Verification items for the finished model (mm, model axes). Coordinates: 2 decimals unless noted, no trailing zeros. Order: outer loops, then holes, each group sorted by start corner. A loop starts at its lowest first (then second) coordinate and runs counter-clockwise, first axis right, second up.
Q1. Depth check by flat-ended pin: P1, Ø8, axis at x = 25, z = 30, coming from the -Y side. Enter the tip coordinate at first touch or a pass-through.
Q2. Draft check along X on faces 1 (the flat face through (30, -2, 81)), 2 (the cylindrical face through (46.15, -1.01, 67.78)). Enter one of: pulls with the +X half, pulls with the -X half, needs draft (parallel to the pull), parting line crosses it, or undercut.
Q3. Cross-section at B-B, the plane z = 150. Record the boundary of the cut face in (x, y).
Q4. Cross-section at C-C, the plane y = -0.7. Count the separate pieces of the cut face and the enclosed holes in it, and give its area (3 significant figures).
Q5. Cross-section at A-A, the plane x = 35. Record the boundary of the cut face in (y, z), and give its area (3 significant figures).
Q6. Thickness scan on line 1 (Z direction, x = 5, y = -0.85); line 2 (Z direction, x = 15, y = -0.55). Record the ranges inside material, lowest first.
from build123d import *

# Parameters (mm, degrees)
SKETCH_W                     = 60
SKETCH_H                     = 160
PAD_DEPTH                    = 2
SKETCH001_R                  = 2.5
POCKET_DEPTH                 = 343.784557
SKETCH001_LINEARPATTERN_2_R  = 2.5
POCKET_LINEARPATTERN_2_DEPTH = 343.784557
SKETCH001_LINEARPATTERN_3_R  = 2.5
POCKET_LINEARPATTERN_3_DEPTH = 343.784557
LINEARPATTERN001_COUNT       = 4
LINEARPATTERN001_PITCH       = 40


with BuildPart() as part:
    # Sketch → Pad (new body)
    with BuildSketch(Plane.XZ):
        with Locations((30, 80)):
            Rectangle(SKETCH_W, SKETCH_H)
    extrude(amount=PAD_DEPTH)

    # Sketch001 (on Face6 of Pad) → Pocket (cut, through all)
    with BuildSketch(Plane.XZ.offset(2)):
        with Locations((15, 12)):
            Circle(SKETCH001_R)
        with Locations((5, 30)):
            Circle(SKETCH001_R)
    pocket = extrude(amount=-POCKET_DEPTH, mode=Mode.SUBTRACT)

    # Sketch001 LinearPattern 2 → Pocket LinearPattern 2 (cut, through all)
    with BuildSketch(Plane(origin=(20, -2, 0), x_dir=(1, 0, 0), z_dir=(0, -1, 0))):
        with Locations((15, 12)):
            Circle(SKETCH001_LINEARPATTERN_2_R)
        with Locations((5, 30)):
            Circle(SKETCH001_LINEARPATTERN_2_R)
    pocket_linearpattern_2 = extrude(amount=-POCKET_LINEARPATTERN_2_DEPTH, mode=Mode.SUBTRACT)

    # Sketch001 LinearPattern 3 → Pocket LinearPattern 3 (cut, through all)
    with BuildSketch(Plane(origin=(40, -2, 0), x_dir=(1, 0, 0), z_dir=(0, -1, 0))):
        with Locations((15, 12)):
            Circle(SKETCH001_LINEARPATTERN_3_R)
        with Locations((5, 30)):
            Circle(SKETCH001_LINEARPATTERN_3_R)
    pocket_linearpattern_3 = extrude(amount=-POCKET_LINEARPATTERN_3_DEPTH, mode=Mode.SUBTRACT)

    # LinearPattern001: Pocket, Pocket LinearPattern 2, Pocket LinearPattern 3 ×4
    with Locations(*[(0, 0, i * LINEARPATTERN001_PITCH) for i in range(1, LINEARPATTERN001_COUNT)]):
        add(pocket, mode=Mode.SUBTRACT)
        add(pocket_linearpattern_2, mode=Mode.SUBTRACT)
        add(pocket_linearpattern_3, mode=Mode.SUBTRACT)


solid = part.part
Check values:
1. P1: stops at y = -2
2. face 1: needs draft
2. face 2: undercut
3. outline: (0, -2) - (2.5, -2) - (2.5, 0) - (0, 0) - close; (7.5, -2) - (22.5, -2) - (22.5, 0) - (7.5, 0) - close; (27.5, -2) - (42.5, -2) - (42.5, 0) - (27.5, 0) - close; (47.5, -2) - (60, -2) - (60, 0) - (47.5, 0) - close
4. separate pieces: 1
4. enclosed holes: 24
4. area: 9,130 mm2
5. outline: (-2, 0) - (0, 0) - (0, 9.5) - (-2, 9.5) - close; (-2, 14.5) - (0, 14.5) - (0, 49.5) - (-2, 49.5) - close; (-2, 54.5) - (0, 54.5) - (0, 89.5) - (-2, 89.5) - close; (-2, 94.5) - (0, 94.5) - (0, 129.5) - (-2, 129.5) - close; (-2, 134.5) - (0, 134.5) - (0, 160) - (-2, 160) - close
5. area: 280 mm2
6. line 1: z = 0 to 27.5, 32.5 to 67.5, 72.5 to 107.5, 112.5 to 147.5, 152.5 to 160
6. line 2: z = 0 to 9.5, 14.5 to 49.5, 54.5 to 89.5, 94.5 to 129.5, 134.5 to 160
